Source: CAD feature listing. Evaluate the final solid. Frame: model axes, mm. A direction names the side the tool comes from. Coordinates: 2 decimals unless noted, no trailing zeros. Order: outer loops, then holes, each group sorted by start corner. A loop starts at its lowest first (then second) coordinate and runs counter-clockwise, first axis right, second up.
Item 1: Section A-A on z = -12. Return the cut outline in (x, y).
Item 2: Section B-B on z = 24.5. Return the cut outline in (x, y).
Item 3: Contact query for flat-ended pins moving along their axis: P1, Ø6, axis at y = -17.5, z = -26.5, coming from the +X side; P2, Ø1, axis at x = 25.5, z = -7.5, coming from the +Y side; P3, Ø2, axis at x = 12.5, z = 28.5, coming from the -Y side; P4, Ø5, axis at y = 33, z = 38.5, coming from the -X side. Output: stop coordinate, or through.
Item 4: Mould query, pull axis Z, two halves, no side actions, for faces 3 (the conical face through (5.04, -22.69, 6.79)), 4 (the cylindrical face through (42.1, 1.85, -36.75)), 5 (the flat face through (1, 1, -40.96)). Classes: released by +Z, released by -Z, zero draft, split by the parting line, or undercut.
Item 5: Ray query, line 1 (Z direction, x = 14.5, y = -8); line 2 (Z direction, x = -22.5, y = 20); line 3 (Z direction, x = 3.5, y = -28). Return the intervals inside material, ascending.
Item 6: Reachability of faces 1 (the cylindrical face through (6.24, -28.08, -12.15)), 2 (the conical face through (6.59, -29.67, 44.52)) from +Z, -Z, +X, -X, +Y, -Y: full face, straight path, thin tool, end or side. Return the list, or none.
from build123d import *


# Not quite as in the source:
# - a feature names something its author has since deleted; it is built from what else it names


with BuildPart() as f1:
    # F0 (on Front) → F1 (revolve)
    with BuildSketch(Plane.XZ):
        with BuildLine():
            Line((-28.766008094, 0), (-28.766008094, -23.9662192762))
            Line((-28.766008094, -23.9662192762), (-42.1394705772, -32.4264727533))
            Line((-42.1394705772, -32.4264727533), (-42.1394705772, -40.9603528678))
            Line((-42.1394705772, -40.9603528678), (0, -40.9603528678))
            Line((0, -40.9603528678), (0, 65.5130892992))
            ThreePointArc((0, 65.5130892992), (-11.6659559175, 59.2375527161), (-10.0377807394, 46.0912249982))
            Line((-10.0377807394, 46.0912249982), (-30.3286965936, 46.1038053036))
            Line((-30.3286965936, 46.1038053036), (-30.560169369, 40.5484326184))
            Line((-30.560169369, 40.5484326184), (-22.8700842708, 31.5248221159))
            Line((-22.8700842708, 31.5248221159), (-22.8700842708, 7.2474917397))
            Line((-22.8700842708, 7.2474917397), (-28.766008094, 0))
        make_face()
    revolve(axis=Axis((0, 0, 12.2763682157), (0, 0, -1)))


solid = f1.part
Answer list:
1. outline: circle Ø57.53 at (0, 0)
2. outline: circle Ø45.74 at (0, 0)
3. P1: stops at x = 33.4
3. P2: stops at y = 14.23
3. P3: stops at y = -19.77
3. P4: passes through
4. face 3: undercut
4. face 4: zero draft
4. face 5: released by -Z
5. line 1: z = -40.96 to 46.1
5. line 2: z = -40.96 to -24.81, 40.01 to 46.1
5. line 3: z = -40.96 to 0.67, 37.8 to 46.1
6. face 1: none
6. face 2: +Z
